Work out the finished part from the listing and answer in its coordinate system (mm). Coordinates: 2 decimals unless noted, no trailing zeros. Write each loop counter-clockwise with the first axis right and the second up, starting at its lowest first coordinate (ties: lowest second). Pieces come first, ordered by that corner, then holes. Notation, with made-up numbers: M 10,-6 L 42,-6 A9 cw 42,3 Z; hole C 39,47.25 d1. An arc over 180 degrees is marked long. Use CSV: the item, a comma, the result in double quotes.
from build123d import *

# Parameters (mm, degrees)
F0_W     = 9
F0_H     = 9
F0_R     = 3
F0_R_2   = 18
F0_R_3   = 9
F0_R_4   = 4.5
F1_DEPTH = 25


with BuildPart() as f1:
    # F0 (on Top) → F1 (new body)
    with BuildSketch(Plane.XY):
        Polygon((-52.684808, 173.482456), (-58.684808, 173.482456), (-58.684808, 24.982456), (-9.184808, 24.982456), (-9.184808, 50.482456), (59.815192, 50.482456), (59.815192, 86.982456), (59.815192, 173.482456), (7.315192, 173.482456), align=None)
        with Locations((-49.684808, 33.980483)):
            Rectangle(F0_W, F0_H, mode=Mode.SUBTRACT)
        with Locations((-33.934808, 33.980483)):
            Rectangle(F0_W, F0_H, mode=Mode.SUBTRACT)
        with Locations((-52.684808, 56.482456)):
            Circle(F0_R, mode=Mode.SUBTRACT)
        with Locations((-18.184808, 33.980483)):
            Rectangle(F0_W, F0_H, mode=Mode.SUBTRACT)
        with Locations((-22.684808, 86.982456)):
            Circle(F0_R_2, mode=Mode.SUBTRACT)
        with Locations((53.815192, 56.482456)):
            Circle(F0_R, mode=Mode.SUBTRACT)
        with Locations((16.315192, 86.982456)):
            Circle(F0_R_3, mode=Mode.SUBTRACT)
        with Locations((41.815192, 86.982456)):
            Circle(F0_R_3, mode=Mode.SUBTRACT)
        with Locations((-31.923011, 116.548747)):
            Circle(F0_R, mode=Mode.SUBTRACT)
        with BuildLine():
            Line((-49.618921, 127.439418), (-49.684808, 151.439328))
            Line((-49.684808, 151.439328), (-25.684899, 151.505215))
            Line((-25.684899, 151.505215), (-25.434899, 151.505215))
            ThreePointArc((-25.434899, 151.505215), (-22.783248, 150.406866), (-21.684899, 147.755215))
            Line((-21.684899, 147.755215), (-21.684899, 147.710127))
            ThreePointArc((-21.684899, 147.710127), (-22.783248, 145.058476), (-25.434899, 143.960127))
            Line((-25.434899, 143.960127), (-25.684899, 143.960127))
            Line((-25.684899, 143.960127), (-42.098359, 143.960127))
            Line((-42.098359, 143.960127), (-42.118949, 127.460008))
            Line((-42.118949, 127.460008), (-49.618921, 127.439418))
        make_face(mode=Mode.SUBTRACT)
        with BuildLine():
            ThreePointArc((-49.684808, 167.482456), (-54.806129, 165.361135), (-52.684808, 170.482456))
            ThreePointArc((-52.684808, 170.482456), (-50.563488, 169.603776), (-49.684808, 167.482456))
        make_face(mode=Mode.SUBTRACT)
        with BuildLine():
            Line((1.315192, 114.520175), (1.315192, 133.982456))
            Line((1.315192, 133.982456), (1.315192, 135.982456))
            ThreePointArc((1.315192, 135.982456), (3.072551, 140.225096), (7.315192, 141.982456))
            Line((7.315192, 141.982456), (8.315192, 141.982456))
            ThreePointArc((8.315192, 141.982456), (12.557832, 140.225096), (14.315192, 135.982456))
            Line((14.315192, 135.982456), (14.315192, 132.982456))
            Line((14.315192, 132.982456), (14.315192, 112.520175))
            ThreePointArc((14.315192, 112.520175), (12.557832, 108.277534), (8.315192, 106.520175))
            Line((8.315192, 106.520175), (7.315192, 106.520175))
            ThreePointArc((7.315192, 106.520175), (3.072551, 108.277534), (1.315192, 112.520175))
            Line((1.315192, 112.520175), (1.315192, 114.520175))
        make_face(mode=Mode.SUBTRACT)
        with Locations((33.959863, 112.520175)):
            Circle(F0_R, mode=Mode.SUBTRACT)
        with Locations((46.291271, 112.520175)):
            Circle(F0_R_4, mode=Mode.SUBTRACT)
        with Locations((53.815192, 167.482456)):
            Circle(F0_R, mode=Mode.SUBTRACT)
    extrude(amount=F1_DEPTH)


solid = f1.part
Item 1: The part is cut by section B-B (y = 91.5). Write down the section's boundary in (x, z).
Answer:
outline,"M -58.68,0 L -40.11,0 L -40.11,25 L -58.68,25 Z; M -5.26,0 L 8.53,0 L 8.53,25 L -5.26,25 Z; M 24.1,0 L 34.03,0 L 34.03,25 L 24.1,25 Z; M 49.6,0 L 59.82,0 L 59.82,25 L 49.6,25 Z"
Item 2: Given pin 1 (7 mm diameter, centred on y = 35.5, z = 12.5, fed in from +X); pin 2 (5 mm diameter, centred on x = 53.82, y = 167.48, fed in from -Z); pin 3 (8 mm diameter, centred on x = 45, z = 11.5, fed in from -Y), each flat-ended and moving along its own axis, determine where each tip first touches the part or whether it passes through.
Answer:
pin 1,"stops at x = -9.18"
pin 2,"passes through"
pin 3,"stops at y = 50.48"
Item 3: The part is cut by section D-D (x = 18.5). Write down the section's boundary in (y, z).
Answer:
outline,"M 50.48,0 L 78.25,0 L 78.25,25 L 50.48,25 Z; M 95.71,0 L 173.48,0 L 173.48,25 L 95.71,25 Z"
Item 4: Consider probe 1 along X at (y, z) = (36.5, 17); probe 2 along Y at (x, z) = (-44, 6); probe 3 along Y at (x, z) = (-52, 1.75). Determine where each line is inside the solid, lowest interval first.
Answer:
probe 1,"x = -58.68 to -54.18, -45.18 to -38.43, -29.43 to -22.68, -13.68 to -9.18"
probe 2,"y = 24.98 to 127.45, 151.45 to 173.48"
probe 3,"y = 24.98 to 29.48, 38.48 to 53.56, 59.4 to 164.56, 170.4 to 173.48"
Item 5: The part is cut by section C-C (x = -31.5). Write down the section's boundary in (y, z), then the cut area to 3 significant figures.
Answer:
outline,"M 24.98,0 L 29.48,0 L 29.48,25 L 24.98,25 Z; M 38.48,0 L 71.29,0 L 71.29,25 L 38.48,25 Z; M 102.68,0 L 113.58,0 L 113.58,25 L 102.68,25 Z; M 119.52,0 L 143.96,0 L 143.96,25 L 119.52,25 Z; M 151.49,0 L 173.48,0 L 173.48,25 L 151.49,25 Z"
area,"2,370 mm2"
Item 6: For a pull along Y with two mould halves and no side action, classify faces 1 (the face through (-34, 24.982, 12)), 2 (the face through (0, 100, 25)), 3 (the face through (-18, 29.48, 12)), 4 (the face through (1, 173.482, 12)) as released by +Y, released by -Y, zero draft, split by the parting line, or undercut.
Answer:
face 1,"released by -Y"
face 2,"zero draft"
face 3,"undercut"
face 4,"released by +Y"
Item 7: The part is cut by section A-A (y = 131). Write down the section's boundary in (x, z).
Answer:
outline,"M -58.68,0 L -49.63,0 L -49.63,25 L -58.68,25 Z; M -42.11,0 L 1.32,0 L 1.32,25 L -42.11,25 Z; M 14.32,0 L 59.82,0 L 59.82,25 L 14.32,25 Z"
